Work out the finished part from the listing and answer in its coordinate system (mm). A direction names the side the tool comes from. Round coordinates to 2 decimals unless told otherwise and drop trailing zeros. Loops run counter-clockwise (first coordinate to the right, second up) from the corner with the lowest first, then second, coordinate; pieces in that order, holes last.
```python
from build123d import *

# Parameters (mm, degrees)
F1_DEPTH = 3


with BuildPart() as f1:
    # F0 (on Front) → F1 (new body)
    with BuildSketch(Plane.XZ):
        Polygon((0, 3.5), (0, 0), (0, -3.5), (3, -3.5), (3, -13.5), (0, -13.5), (0, -20.5), (7, -20.5), (7, -23.5), (17, -23.5), (17, -20.5), (19.5, -20.5), (19.5, -14.5), (17.5, -14.5), (17.5, -12.5), (19.5, -12.5), (19.5, -8.5), (21.5, -8.5), (21.5, -12.5), (23.5, -12.5), (23.5, -14.5), (21.5, -14.5), (21.5, -20.5), (24, -20.5), (24, -23.5), (34, -23.5), (34, -20.5), (41, -20.5), (41, -13.5), (38, -13.5), (38, -3.5), (41, -3.5), (41, 0), (41, 3.5), (38, 3.5), (38, 13.5), (41, 13.5), (41, 20.5), (34, 20.5), (34, 23.5), (24, 23.5), (24, 20.5), (21.5, 20.5), (21.5, 14.5), (23.5, 14.5), (23.5, 12.5), (21.5, 12.5), (21.5, 8.5), (19.5, 8.5), (19.5, 12.5), (17.5, 12.5), (17.5, 14.5), (19.5, 14.5), (19.5, 20.5), (17, 20.5), (17, 23.5), (7, 23.5), (7, 20.5), (0, 20.5), (0, 13.5), (3, 13.5), (3, 3.5), align=None)
    extrude(amount=F1_DEPTH)


solid = f1.part
```
1. Consider probe 1 along Z at (x, y) = (22.5, -1.1); probe 2 along X at (y, z) = (-2.85, -15.5); probe 3 along X at (y, z) = (-1.6, -9.5). Determine where each line is inside the solid, lowest interval first.
Answer key:
probe 1: z = -20.5 to -14.5, -12.5 to 12.5, 14.5 to 20.5
probe 2: x = 0 to 19.5, 21.5 to 41
probe 3: x = 3 to 19.5, 21.5 to 38
2. Given pin 1 (1.5 mm diameter, centred on x = 39, y = -2, fed in from +Z); pin 2 (0.9 mm diameter, centred on y = -1, z = 8.5, fed in from -X); pin 3 (0.6 mm diameter, centred on x = 19, y = -2, fed in from -Z), each flat-ended and moving along its own axis, determine where each tip first touches the part or whether it passes through.
Answer key:
pin 1: stops at z = 20.5
pin 2: stops at x = 3
pin 3: stops at z = -20.5
3. Determine the mould class of faces 5 (the face through (19.5, -1, 10)), 6 (the face through (17, -1, 22)), 7 (the face through (40, -1, -13.5)), 8 (the face through (3, -1, 9)) for opening direction X: +X half, -X half, draft (parallel to the pull), parting line (faces both ways), or undercut.
Answer key:
face 5: undercut
face 6: undercut
face 7: draft
face 8: -X half
4. Find section B-B (z = -8). Write down the section's boundary in (x, y), then the cut area to 3 significant figures.
Answer key:
outline: (3, -3) - (38, -3) - (38, 0) - (3, 0) - close
area: 105 mm2
5. Which of the six approach directions +Z, -Z, +X, -X, +Y, -Y give full straight-line access (tool end or side, diameter ignored) to faces 1 (the face through (34, -1, 22)), 2 (the face through (37, -1, -20.5)), 3 (the face through (23, -1, -20.5)), 4 (the face through (21.5, -1, 11))?
Answer key:
face 1: +Z, +X, +Y, -Y
face 2: -Z, +X, +Y, -Y
face 3: -Z, +Y, -Y
face 4: +Z, +Y, -Y
6. Find section A-A (z = -13). Write down the section's boundary in (x, y), then the cut area to 3 significant figures.
Answer key:
outline: (3, -3) - (17.5, -3) - (17.5, 0) - (3, 0) - close; (23.5, -3) - (38, -3) - (38, 0) - (23.5, 0) - close
area: 87.0 mm2
